Autodesk Inventor part; units mm, degrees
ref_plane "YZ Plane" through (0, 0, 0) normal (1, 0, 0) x (0, 1, 0)
ref_plane "XZ Plane" through (0, 0, 0) normal (0, 1, 0) x (-1, 0, 0)
ref_plane "XY Plane" through (0, 0, 0) normal (0, 0, 1) x (1, 0, 0)
sketch "スケッチ1" plane through (0, 0, 0) normal (0, 1, 0) x (-1, 0, 0)
  line L0 (26, 0) -> (0, 0)
  line L1 (0, 0) -> (0, -15)
  line L2 (0, -15) -> (26, -15)
  line L3 (26, -15) -> (26, 0)
  line L4 (36.4849, 5.9511) -> (26, -20)
  line L5 (26, -20) -> (0, -20)
  line L6 (0, -20) -> (-10.4849, 5.9511)
  arc A0 (36.4849, 5.9511) -> (-10.4849, 5.9511) centre (13, -20) ccw
  line L7 (0, 0) -> (26, -15)
  line L8 (0, -15) -> (26, 0)
  line L9 (4, -2.3077) -> (22, -2.3077)
  line L10 (22, -2.3077) -> (22, -12.6923)
  line L11 (22, -12.6923) -> (4, -12.6923)
  line L12 (4, -12.6923) -> (4, -2.3077)
  circle A1 centre (4, -2.3077) radius 0.8
  circle A2 centre (4, -12.6923) radius 0.8
  circle A3 centre (22, -2.3077) radius 0.8
  circle A4 centre (22, -12.6923) radius 0.8
  circle A5 centre (13, -7.5) radius 0.8
  point P0 (22.6929, -13.0921)
  point P1 (21.2, -12.6923)
  dimension "d0" = 26
  dimension "d1" = 15
  dimension "d4" = 22
  dimension "d5" = 22
  dimension "d6" = 5
  dimension "d7" = 35
  dimension "d23" = 4
  dimension "d24" = 1.6
  dimension "d25" = 1.6
  dimension "d26" = 1.6
  dimension "d27" = 1.6
  dimension "d32" = 1.6
extrude "押し出し1" add sketch "スケッチ1" along normal blind 4 contours L8 A3 L9 A1 L7 L0 | L3 L7 A4 L10 A3 L8 | L7 A1 L12 A2 L8 L1 | L2 L8 A2 L11 A4 L7 | A3 L10 L8 | L8 L9 A3 | A1 L9 L7 | L7 L12 A1 | L10 A3 L8 | L8 A3 L9 | A3 L8 A5 L7 A1 L9 | L9 A1 L7 | L7 A1 L12 | A1 L7 A5 L8 A2 L12 | L11 A2 L8 A5 L7 A4 | A3 L10 A4 L7 A5 L8 | L4 L5 L6 A0
sketch "スケッチ2" plane through (0, 0, 0) normal (0, -1, 0) x (1, 0, 0)
  arc A0 (-29.9016, 8.3432) -> (-34.0957, 5.3766) centre (-13, -20) ccw
  arc A1 (10.4849, 5.9511) -> (-36.4849, 5.9511) centre (-13, -20) ccw
  arc A2 (8.0957, 5.3766) -> (3.9016, 8.3432) centre (-13, -20) ccw
  line L0 (8.0957, 5.3766) -> (-1.349, -18)
  line L1 (-29.9016, 8.3432) -> (-19.2583, -18)
  line L2 (-34.0957, 5.3766) -> (-24.651, -18)
  line L3 (10.4849, 5.9511) -> (0, -20)
  line L4 (-26, -20) -> (-36.4849, 5.9511)
  line L5 (3.9016, 8.3432) -> (-6.7417, -18)
  line L6 (-24.651, -18) -> (-19.2583, -18)
  line L7 (0, -20) -> (-26, -20)
  line L8 (-6.7417, -18) -> (-1.349, -18)
  circle A3 centre (-4, -12.6923) radius 0.8
  circle A4 centre (-22, -12.6923) radius 0.8
  circle A5 centre (-4, -12.6923) radius 2.5
  circle A6 centre (-22, -12.6923) radius 2.5
  circle A7 centre (-13, -7.5) radius 0.8
  circle A8 centre (-13, -7.5) radius 2.5
  arc A9 (-22.5806, 11.5787) -> (-29.9016, 8.3432) centre (-13, -20) ccw
  arc A10 (3.9016, 8.3432) -> (-3.4194, 11.5787) centre (-13, -20) ccw
  line L9 (-22.5806, 11.5787) -> (-19.3484, 3.5787)
  line L10 (-19.3484, 3.5787) -> (-26.7659, 0.5818)
  line L11 (-3.4194, 11.5787) -> (-6.6516, 3.5787)
  line L12 (-6.6516, 3.5787) -> (0.7659, 0.5818)
  point P0 (-22.3998, -10.2245)
  point P1 (-20.5733, -14.7452)
  point P2 (-5.4267, -14.7452)
  point P3 (-3.6002, -10.2245)
  dimension "d10" = 2
  dimension "d11" = 2
  dimension "d14" = 2
  dimension "d15" = 2
  dimension "d16" = 5
  dimension "d17" = 2
  dimension "d18" = 2
  dimension "d19" = 5
  dimension "d29" = 5
  dimension "d30" = 5
  dimension "d33" = 5
  dimension "d50" = 8
  dimension "d51" = 8
  dimension "d52" = 8
  dimension "d53" = 8
extrude "押し出し2" add sketch "スケッチ2" along normal blind 1 contours L3 L7 L4 A1
fillet "フィレット1" radius 0.5 14 edges at (3.3734, -1, -6.3117) (2.6485, -1, 9.0538) (-6.0842, -1, -16.3726) (-1.4172, -1, -4.8213) (-4.0454, -1, -18) (-19.9158, -1, -16.3726) (-24.5828, -1, -4.8213) (-21.9546, -1, -18) (-29.3734, -1, -6.3117) (-28.6485, -1, 9.0538) (-5.0355, -1, 7.5787) (-2.9429, -1, 2.0802) (-20.9645, -1, 7.5787) (-23.0571, -1, 2.0802)
extrude "押し出し3" cut sketch "スケッチ2" against normal blind 1 contours A6 L1 A4 | L1 A4 A6 | A4 L1 | L1 A4 | A5 L5 A3 | L5 A3 A5 | A3 L5 | L5 A3 | A8
fillet "フィレット2" radius 2 4 edges at (10.4849, 1.5, 5.9511) (0, 1.5, -20) (-26, 1.5, -20) (-36.4849, 1.5, 5.9511)
equation "\"d5\" = d4"
properties part number "toe_sole_front"
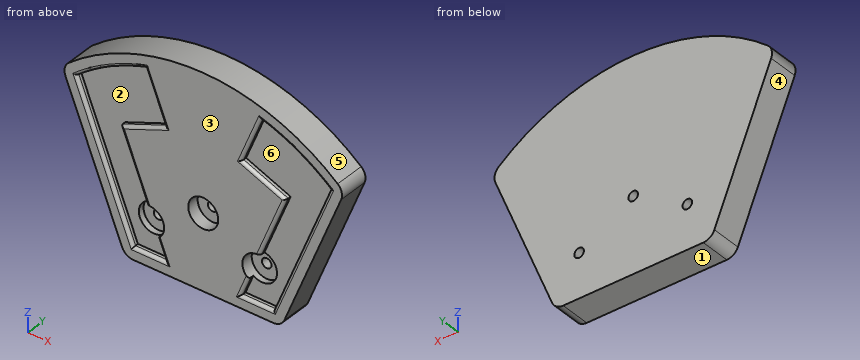
Could you check a few things on this model? Use its own coordinates, in mm. Face numbers are marked on the shaded views. A direction names the side the tool comes from. Give positions to 0.01 mm unless a question says otherwise; leave off trailing zeros. Loops run counter-clockwise (first coordinate to the right, second up) from the corner with the lowest first, then second, coordinate; pieces in that order, holes last. Notation, with made-up numbers: (71, -35) - (116, -35) arc R26 ccw to (116, -13) - close; hole circle Ø11 at (-9, -22). An arc over 180 degrees is marked (long way). Answer in a Markdown table with one row per item. Add a question column.
Q1. Which directions (+Z, -Z, +X, -X, +Y, -Y) give clear straight access to the entire face, cutting with the end or side of a thin tool? Please do the marked faces 1 and 2.
Q2. If we section it at A-A (x = -13): List the corners of the cut face in (y, z) for me, plus the area to 3 significant figures.
Q3. Please list where these lines run through material, in increasing order: L1, parallel to Z at x = -22, y = -0.5; L2, parallel to Z at x = -13, y = 0.45; L3, parallel to Z at x = -13, y = 2.1. Write a range as from..to.
Q4. For pin 1 (1 mm diameter, centred on x = -8, y = 3.5, fed in from +Z); pin 2 (2.5 mm diameter, centred on x = -13, z = -7.5, fed in from -Y); pin 3 (2 mm diameter, centred on x = -30.5, y = 1, fed in from -Z); pin 4 (1.3 mm diameter, centred on x = -22, z = -12.69, fed in from +Y), each with a flat end and sliding along its axis, tell me the tip position at first contact or that it passes through.
Q5. We'd pull the mould along X, two halves only. Please class the marked faces 3, 4, 5 and 6: +X half, -X half, draft (parallel to the pull), parting line (faces both ways), or undercut.
Q6. If we section it at B-B (y = 3.3): List the corners of the cut face in (x, z) for me.
The answers:
| question | item | result |
|---|---|---|
| 1 | face 1 | -Z, +X, -X, +Y, -Y |
| 1 | face 2 | -Y |
| 2 | outline | (-1, -20) - (4, -20) - (4, -8.3) - (1, -8.3) - (1, -10) - (-1, -10) - close; (-1, -5) - (1, -5) - (1, -6.7) - (4, -6.7) - (4, 15) - (-1, 15) - close |
| 2 | area | 160 mm^2 |
| 3 | L1 | z = -20..-18, -10.19..2.51, 10.14..13.82 |
| 3 | L2 | z = -20..-10, -5..15 |
| 3 | L3 | z = -20..-8.3, -6.7..15 |
| 4 | pin 1 | stops at z = 14.71 |
| 4 | pin 2 | stops at y = 1 |
| 4 | pin 3 | stops at z = -11.34 |
| 4 | pin 4 | passes through |
| 5 | face 3 | draft |
| 5 | face 4 | -X half |
| 5 | face 5 | parting line |
| 5 | face 6 | undercut |
| 6 | outline | (-35.95, 4.63) - (-26.51, -18.75) arc R2 ccw to (-24.65, -20) - (-1.35, -20) arc R2 ccw to (0.51, -18.75) - (9.95, 4.63) arc R2 ccw to (9.37, 6.91) arc R35 ccw to (-35.37, 6.91) arc R2 ccw to start; hole circle Ø1.6 at (-22, -12.69); hole circle Ø1.6 at (-13, -7.5); hole circle Ø1.6 at (-4, -12.69) |
